Model file for the job. Use its own axes, mm. Round coordinates to 2 decimals unless told otherwise and drop trailing zeros. Loops run counter-clockwise (first coordinate to the right, second up) from the corner with the lowest first, then second, coordinate; pieces in that order, holes last. Notation, with made-up numbers: (36, -9) -> (57, -9) arc R23 cw to (57, 7) -> close; hole circle Ø8 at (43, -35). An arc over 180 degrees is marked (long way). Use a Markdown table: item, result.
from build123d import *

# Parameters (mm, degrees)
F0_W     = 50.8
F0_H     = 50.8
F1_DEPTH = 25.4
F4_R     = 5.08
F5_DEPTH = 25.4


with BuildPart() as f1:
    # F0 (on Front) → F1 (new body, symmetric)
    with BuildSketch(Plane.XZ):
        Rectangle(F0_W, F0_H)
    extrude(amount=F1_DEPTH, both=True)

    # F2 (on Front) → F3 (revolve, cut)
    with BuildSketch(Plane.XZ):
        with BuildLine():
            Line((0, -12.7), (0, 12.7))
            ThreePointArc((0, 12.7), (-12.7, 0), (0, -12.7))
        make_face()
    revolve(axis=Axis((0, 0, 0), (0, 0, -1)), mode=Mode.SUBTRACT)

    # F4 (on face) → F5 (cut)
    with BuildSketch(Plane.XZ.offset(25.4)):
        Circle(F4_R)
    extrude(amount=-F5_DEPTH, mode=Mode.SUBTRACT)


solid = f1.part
Q1. Flat gauge pin, fed straight in: pin 1 (9 mm diameter, centred on x = 0, z = 0, fed in from -Y). Where does the tip first touch, or does it go through?
Results list:
| item | result |
|---|---|
| pin 1 | stops at y = 11.88 |
Q2. Band-saw the part on B-B, the plane z = 0. Give the cut face in (x, y), plus the area to 3 significant figures.
Results list:
| item | result |
|---|---|
| outline | (-25.4, -25.4) -> (-5.08, -25.4) -> (-5.08, -11.64) arc R12.7 cw (long way) to (5.08, -11.64) -> (5.08, -25.4) -> (25.4, -25.4) -> (25.4, 25.4) -> (-25.4, 25.4) -> close |
| area | 1,940 mm² |
Q3. Drill centre lines: L1, parallel to X at y = -14.5, z = 0; L2, parallel to Z at x = -1, y = -2.5. Where is each one in solid material? Low to high. Write a range as from..to.
Results list:
| item | result |
|---|---|
| L1 | x = -25.4..-5.08, 5.08..25.4 |
| L2 | z = -25.4..-12.41, 12.41..25.4 |
Q4. Pull direction X, two halves, no side cores. Call faces 1 (the face through (-25.4, 0, 0)), 2 (the face through (0, 25.4, 0)), 3 (the face through (25.4, 0, 0)), 4 (the face through (-0.661, -18.616, 5.037)): released by +X, released by -X, zero draft, split by the parting line, or undercut.
Results list:
| item | result |
|---|---|
| face 1 | released by -X |
| face 2 | zero draft |
| face 3 | released by +X |
| face 4 | undercut |
Q5. Band-saw the part on C-C, the plane y = 4. Give the cut face in (x, z).
Results list:
| item | result |
|---|---|
| outline | (-25.4, -25.4) -> (25.4, -25.4) -> (25.4, 25.4) -> (-25.4, 25.4) -> close; hole circle Ø24.11 at (0, 0) |
Q6. Band-saw the part on A-A, the plane x = 0. Give the cut face in (y, z).
Results list:
| item | result |
|---|---|
| outline | (-25.4, -25.4) -> (25.4, -25.4) -> (25.4, 25.4) -> (-25.4, 25.4) -> (-25.4, 5.08) -> (-11.64, 5.08) arc R12.7 cw (long way) to (-11.64, -5.08) -> (-25.4, -5.08) -> close |
Q7. Band-saw the part on D-D, the plane z = -10.5. Give the cut face in (x, y).
Results list:
| item | result |
|---|---|
| outline | (-25.4, -25.4) -> (25.4, -25.4) -> (25.4, 25.4) -> (-25.4, 25.4) -> close; hole circle Ø14.29 at (0, 0) |
